Check sheet for the modelled part. Datum: model origin and axes. Units: mm. Face numbers are marked on the shaded views. A direction names the side the tool comes from. Coordinates: 2 decimals unless noted, no trailing zeros. Loops run counter-clockwise (first coordinate to the right, second up) from the corner with the lowest first, then second, coordinate; pieces in that order, holes last. Notation, with made-up numbers: (66.5, -2) - (84.5, -2) arc R24 ccw to (84.5, 22) - close; hole circle Ø11 at (14.25, -36.5). An arc over 180 degrees is marked (long way). Use a Markdown table: item, result. Add a question column.
1) Tool access check on the marked faces 4 and 5. Record the directions out of +Z, -Z, +X, -X, +Y, -Y that give a thin tool (end or side, any length) a straight path to the whole face; none if there is none.
2) Sectioned sample at D-D, the plane y = 12. Enter the section's corners in (x, z).
3) Sectioned sample at B-B, the plane z = -5.5. Enter the section's corners in (x, y), then the cut area to 3 significant figures.
4) Draft check along Z on the marked faces 1, 2 and 3. Enter one of: pulls with the +Z half, pulls with the -Z half, needs draft (parallel to the pull), parting line crosses it, or undercut.
5) Sectioned sample at C-C, the plane x = 2. Enter the section's corners in (y, z).
6) Go/stop test with flat-tipped pins: P1, Ø1.6, axis at y = 1, z = -9.5, coming from the +X side; P2, Ø7, axis at x = 2.5, y = 18, coming from the -Z side; P3, Ø4.5, axis at x = -4.5, z = 10.5, coming from the +Y side. Record where each tip stops, or that it passes through.
7) Thickness scan on line 1 (Z direction, x = -0.25, y = 30); line 2 (Y direction, x = -2, z = 1.25); line 3 (X direction, y = 1.2, z = 10). Record the ranges inside material, lowest first.
8) Sectioned sample at A-A, the plane x = -5. Enter the section's corners in (y, z).
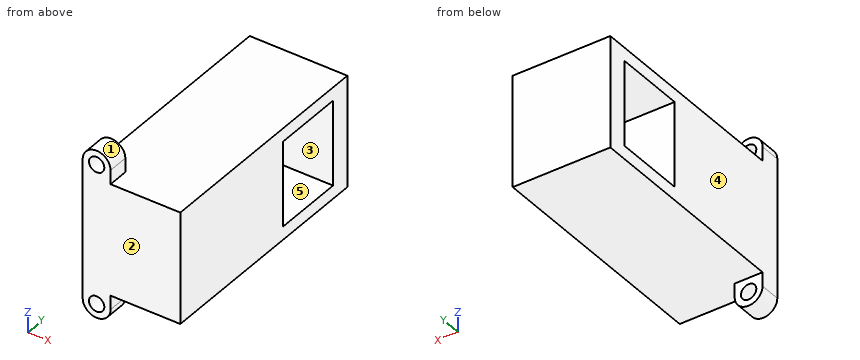
from build123d import *

# Parameters (mm, degrees)
SKETCH_1_W               = 14
SKETCH_1_H               = 16
EXTRUDE_1_DEPTH          = 34
CUT_EXTRUDE_1_DEPTH      = 36.623026261
CUT_EXTRUDE_1_DEPTH_BACK = 36.623026261
SKETCH_2_W               = 12.2
SKETCH_2_H               = 10.2
SKETCH_3_R               = 1.1
EXTRUDE_2_DEPTH          = 3


with BuildPart() as part:
    # 草图1 → 凸台-拉伸1 (new body)
    with BuildSketch(Plane(origin=(0, 0, 0), x_dir=(1, 0, 0), z_dir=(0, 1, 0))):
        Rectangle(SKETCH_1_W, SKETCH_1_H)
    extrude(amount=EXTRUDE_1_DEPTH)

    # 草图2 → 切除-拉伸1 (cut, two sides: drawn at the far end of the back side and taken through both)
    with BuildSketch(Plane(origin=(0, 0, 0), x_dir=(0, 0, -1), z_dir=(1, 0, 0)).offset(-CUT_EXTRUDE_1_DEPTH_BACK)):
        with Locations((0, 26)):
            Rectangle(SKETCH_2_W, SKETCH_2_H)
    extrude(amount=CUT_EXTRUDE_1_DEPTH + CUT_EXTRUDE_1_DEPTH_BACK, mode=Mode.SUBTRACT)

    # 草图3 → 凸台-拉伸2 (add)
    with BuildSketch(Plane(origin=(0, 0, 0), x_dir=(1, 0, 0), z_dir=(0, 1, 0))):
        with BuildLine():
            Line((-7, 8), (-7, 10))
            ThreePointArc((-7, 10), (-5, 12), (-3, 10))
            Line((-3, 10), (-3, 8))
            Line((-3, 8), (-7, 8))
        make_face()
        with Locations(Location((-5, 10, 0), (0, 0, 270))):
            Circle(SKETCH_3_R, mode=Mode.SUBTRACT)
    extrude_2 = extrude(amount=EXTRUDE_2_DEPTH)

    # 镜向1: 凸台-拉伸2 across plane
    add(extrude_2.mirror(Plane.XY))


solid = part.part
Solved:
| question | item | result |
|---|---|---|
| 1 | face 4 | +Z, -Z, -X, +Y, -Y |
| 1 | face 5 | +X, -X |
| 2 | outline | (-7, -8) - (7, -8) - (7, 8) - (-7, 8) - close |
| 3 | outline | (-7, 0) - (7, 0) - (7, 20.9) - (-7, 20.9) - close; (-7, 31.1) - (7, 31.1) - (7, 34) - (-7, 34) - close |
| 3 | area | 333 mm2 |
| 4 | face 1 | pulls with the +Z half |
| 4 | face 2 | needs draft |
| 4 | face 3 | undercut |
| 5 | outline | (0, -8) - (34, -8) - (34, 8) - (0, 8) - close; hole (20.9, -6.1) - (31.1, -6.1) - (31.1, 6.1) - (20.9, 6.1) - close |
| 6 | P1 | stops at x = -3 |
| 6 | P2 | stops at z = -8 |
| 6 | P3 | stops at y = 3 |
| 7 | line 1 | z = -8 to -6.1, 6.1 to 8 |
| 7 | line 2 | y = 0 to 20.9, 31.1 to 34 |
| 7 | line 3 | x = -7 to -6.1, -3.9 to -3 |
| 8 | outline | (0, -12) - (3, -12) - (3, -11.1) - (0, -11.1) - close; (0, -8.9) - (3, -8.9) - (3, -8) - (34, -8) - (34, 8) - (3, 8) - (3, 8.9) - (0, 8.9) - close; (0, 11.1) - (3, 11.1) - (3, 12) - (0, 12) - close; hole (20.9, -6.1) - (31.1, -6.1) - (31.1, 6.1) - (20.9, 6.1) - close |
